Read the model definition and answer for the solid it produces. Units are mm, in the model's axes. Face numbers are marked on the shaded views. A direction names the side the tool comes from. Coordinates: 2 decimals unless noted, no trailing zeros. Loops run counter-clockwise (first coordinate to the right, second up) from the corner with the lowest first, then second, coordinate; pieces in that order, holes last. Notation, with made-up numbers: (40.5, 36) - (57.5, 36) arc R22 ccw to (57.5, 49) - close; hole circle Ø9 at (84.25, -13). An arc over 180 degrees is marked (long way). Use one line per item in the form item = value. Start each with the question number.
1) A cutting plane is placed at A-A (x = -20). Give the vertices of the cut face in (y, z), and give its area (3 significant figures).
2) The mould has two halves that part along Z. Classify the marked faces 6, 7, 8 and 9: released by +Z, released by -Z, zero draft, split by the parting line, or undercut.
3) Which of the six approach directions +Z, -Z, +X, -X, +Y, -Y give full straight-line access (tool end or side, diameter ignored) to the marked faces 1, 2, 3, 4 and 5?
4) A cutting plane is placed at B-B (z = 0). Give the vertices of the cut face in (x, y), and give its area (3 significant figures).
5) Consider line 1 (X direction, y = 7.9, z = 0); line 2 (Z direction, x = -10, y = 27.5); line 3 (X direction, y = 2.9, z = 0). Determine where each line is inside the solid, lowest interval first.
6) A cutting plane is placed at C-C (y = 3.5). Give the vertices of the cut face in (x, z), and give its area (3 significant figures).
7) A cutting plane is placed at D-D (y = 27). Give the vertices of the cut face in (x, z).
8) Each of these flat-tipped pins is pushed along its axis until it touches: P1, Ø4, axis at x = -40, z = 0, coming from the -Y side; P2, Ø1.6, axis at y = 10.5, z = 9.5, coming from the +X side; P3, Ø1, axis at x = 2, y = 10, coming from the -Z side; P4, Ø3, axis at x = -22.5, z = -2.5, coming from the +Y side. Where does it stop, or does it pass through?
from build123d import *

# Parameters (mm, degrees)
CROQUIS1_R              = 2.5
SALIENTE_EXTRUIR1_DEPTH = 10
CROQUIS3_R              = 2.5
SALIENTE_EXTRUIR2_DEPTH = 6.9
MATRIZL1_COUNT          = 2
MATRIZL1_PITCH          = 16.9
CROQUIS6_R              = 5
CORTAR_EXTRUIR1_DEPTH   = 4
REDONDEO3_R             = 0.5


with BuildPart() as part:
    # Croquis1 → Saliente-Extruir1 (new body)
    with BuildSketch(Plane(origin=(0, 0, 0), x_dir=(1, 0, 0), z_dir=(0, 1, 0))):
        with BuildLine():
            Line((0, -11.9), (-40, -11.9))
            ThreePointArc((-40, -11.9), (-51.9, 0), (-40, 11.9))
            Line((-40, 11.9), (0, 11.9))
            ThreePointArc((0, 11.9), (11.9, 0), (0, -11.9))
        make_face()
        with Locations(Location((-40, 0, 0), (0, 0, 270))):
            Circle(CROQUIS1_R, mode=Mode.SUBTRACT)
        with Locations(Location((0, 0, 0), (0, 0, 90))):
            Circle(CROQUIS1_R, mode=Mode.SUBTRACT)
    extrude(amount=SALIENTE_EXTRUIR1_DEPTH)

    # Croquis3 → Saliente-Extruir2 (add)
    with BuildSketch(Plane.XY.offset(11.9)):
        with BuildLine():
            Line((-40, 10), (-40, 11))
            Line((-40, 11), (-32.81186088, 24.657464328))
            ThreePointArc((-32.81186088, 24.657464328), (-29.131109594, 28.56080146), (-23.962678656, 30))
            Line((-23.962678656, 30), (-16.037321344, 30))
            ThreePointArc((-16.037321344, 30), (-10.868890406, 28.56080146), (-7.18813912, 24.657464328))
            Line((-7.18813912, 24.657464328), (0, 11))
            Line((0, 11), (0, 10))
            Line((0, 10), (0, 0))
            Line((0, 0), (-40, 0))
            Line((-40, 0), (-40, 10))
        make_face()
        with Locations((-20, 21)):
            Circle(CROQUIS3_R, mode=Mode.SUBTRACT)
    saliente_extruir2 = extrude(amount=-SALIENTE_EXTRUIR2_DEPTH)

    # MatrizL1: Saliente-Extruir2 ×2
    with Locations(*[(0, 0, -i * MATRIZL1_PITCH) for i in range(1, MATRIZL1_COUNT)]):
        add(saliente_extruir2)

    # Croquis6 → Cortar-Extruir1 (cut, symmetric)
    with BuildSketch(Plane(origin=(0, 10, 0), x_dir=(1, 0, 0), z_dir=(0, 1, 0))):
        with Locations(Location((-40, 0, 0), (0, 0, 270))):
            Circle(CROQUIS6_R)
        with Locations(Location((0, 0, 0), (0, 0, 90))):
            Circle(CROQUIS6_R)
    extrude(amount=CORTAR_EXTRUIR1_DEPTH, both=True, mode=Mode.SUBTRACT)

    # Redondeo3
    # the kernel refuses this fillet: 0.5 mm, written as the material it takes off along each edge
    with BuildSketch(Plane(origin=(-40, 10, 0), x_dir=(0, 0, -1), z_dir=(1, 0, 0))) as redondeo3_piece_1:
        with BuildLine():
            CenterArc((5 + REDONDEO3_R, -REDONDEO3_R), REDONDEO3_R, 90, 90)
            Line((5, -REDONDEO3_R), (5, 0))
            Line((5, 0), (5 + REDONDEO3_R, 0))
        make_face()
    revolve(axis=Axis((-40, 10, 0), (0, 1, 0)), revolution_arc=180, mode=Mode.SUBTRACT)
    with BuildSketch(Plane(origin=(-40, 10, 0), x_dir=(0, 0, 1), z_dir=(-1, 0, 0))) as redondeo3_piece_2_section:
        with BuildLine():
            CenterArc((5 + REDONDEO3_R, -REDONDEO3_R), REDONDEO3_R, 90, 90)
            Line((5 + REDONDEO3_R, 0), (5, 0))
            Line((5, 0), (5, -REDONDEO3_R))
        make_face()
    redondeo3_piece_2 = revolve(axis=Axis((-40, 10, 0), (0, 1, 0)), revolution_arc=180, mode=Mode.PRIVATE)
    redondeo3_piece_2 = split(redondeo3_piece_2, bisect_by=Plane(origin=(-34.859999019, 9.859999019, -5), z_dir=(0, 0, 1)), keep=Keep.TOP, mode=Mode.PRIVATE)
    redondeo3_piece_2 = split(redondeo3_piece_2, bisect_by=Plane(origin=(-34.859999019, 9.859999019, 5), z_dir=(0, 0, -1)), keep=Keep.TOP, mode=Mode.PRIVATE)
    add(redondeo3_piece_2, mode=Mode.SUBTRACT)
    with BuildSketch(Plane(origin=(0, 10, 0), x_dir=(0, 0, -1), z_dir=(1, 0, 0))) as redondeo3_piece_3_section:
        with BuildLine():
            CenterArc((5 + REDONDEO3_R, -REDONDEO3_R), REDONDEO3_R, 90, 90)
            Line((5, -REDONDEO3_R), (5, 0))
            Line((5, 0), (5 + REDONDEO3_R, 0))
        make_face()
    redondeo3_piece_3 = revolve(axis=Axis((0, 10, 0), (0, 1, 0)), revolution_arc=180, mode=Mode.PRIVATE)
    redondeo3_piece_3 = split(redondeo3_piece_3, bisect_by=Plane(origin=(-5.140000985, 9.859999015, -5), z_dir=(0, 0, 1)), keep=Keep.TOP, mode=Mode.PRIVATE)
    redondeo3_piece_3 = split(redondeo3_piece_3, bisect_by=Plane(origin=(-5.140000985, 9.859999015, 5), z_dir=(0, 0, -1)), keep=Keep.TOP, mode=Mode.PRIVATE)
    add(redondeo3_piece_3, mode=Mode.SUBTRACT)
    with BuildSketch(Plane(origin=(0, 10, 0), x_dir=(0, 0, 1), z_dir=(-1, 0, 0))) as redondeo3_piece_4:
        with BuildLine():
            CenterArc((5 + REDONDEO3_R, -REDONDEO3_R), REDONDEO3_R, 90, 90)
            Line((5, -REDONDEO3_R), (5, 0))
            Line((5, 0), (5 + REDONDEO3_R, 0))
        make_face()
    revolve(axis=Axis((0, 10, 0), (0, 1, 0)), revolution_arc=180, mode=Mode.SUBTRACT)


solid = part.part
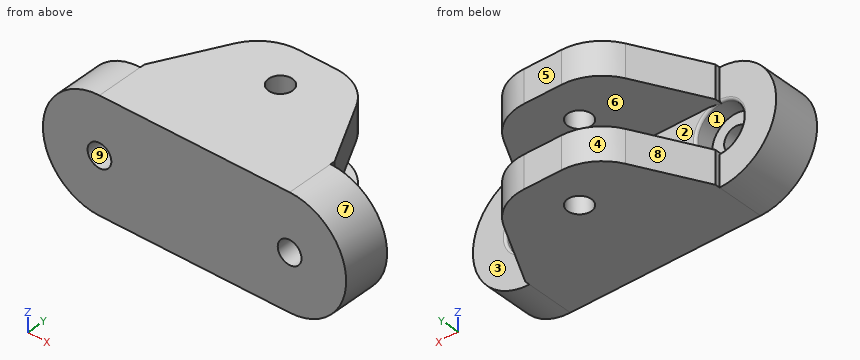
Found:
q1.outline = (0, -11.9) - (18.5, -11.9) - (18.5, -5) - (10, -5) - (10, 5) - (18.5, 5) - (18.5, 11.9) - (0, 11.9) - close; (23.5, -11.9) - (30, -11.9) - (30, -5) - (23.5, -5) - close; (23.5, 5) - (30, 5) - (30, 11.9) - (23.5, 11.9) - close
q1.area = 445 mm^2
q2.face_6 = undercut
q2.face_7 = split by the parting line
q2.face_8 = zero draft
q2.face_9 = undercut
q3.face_1 = +Y
q3.face_2 = +X, -X, +Y
q3.face_3 = +Z, -Z, +X, +Y
q3.face_4 = +Z, -Z, -X, +Y
q3.face_5 = +Z, -Z, +X, -X, +Y
q4.outline = (-51.9, 0) - (-42.5, 0) - (-42.5, 6) - (-45, 6) - (-45, 9.5) arc R0.5 ccw to (-45.5, 10) - (-51.9, 10) - close; (-37.5, 0) - (-2.5, 0) - (-2.5, 6) - (-5, 6) - (-5, 9.5) arc R0.5 ccw to (-5.5, 10) - (-34.5, 10) arc R0.5 ccw to (-35, 9.5) - (-35, 6) - (-37.5, 6) - close; (2.5, 0) - (11.9, 0) - (11.9, 10) - (5.5, 10) arc R0.5 ccw to (5, 9.5) - (5, 6) - (2.5, 6) - close
q4.area = 498 mm^2
q5.line_1 = -51.9 to -45, -35 to -5, 5 to 11.9
q5.line_2 = -11.9 to -5, 5 to 11.9
q5.line_3 = -51.9 to -42.5, -37.5 to -2.5, 2.5 to 11.9
q6.outline = (-40, -11.9) - (0, -11.9) arc R11.9 ccw to (0, 11.9) - (-40, 11.9) arc R11.9 ccw to start; hole circle Ø5 at (-40, 0); hole circle Ø5 at (0, 0)
q6.area = 1,360 mm^2
q7.outline = (-31.1, -11.9) - (-8.9, -11.9) - (-8.9, -5) - (-31.1, -5) - close; (-31.1, 5) - (-8.9, 5) - (-8.9, 11.9) - (-31.1, 11.9) - close
q8.P1 = through
q8.P2 = 7.93
q8.P3 = -11.81
q8.P4 = 10
